Study the drawing (mm; zero at the part's minimum x, y, z) and answer. Coordinates: 2 decimals unless noted, no trailing zeros. Order: outer loops, then holes, each group sorted by start corner. A loop starts at its lowest first (then second) coordinate and runs counter-clockwise, first axis right, second up. Notation, with made-up numbers: (21, -12.5) - (37, -12.5) arc R26 ccw to (37, 6.5) - close; hole circle Ø11 at (-11, 19). An arc over 180 degrees is marked (long way). Write item = value, one per line.
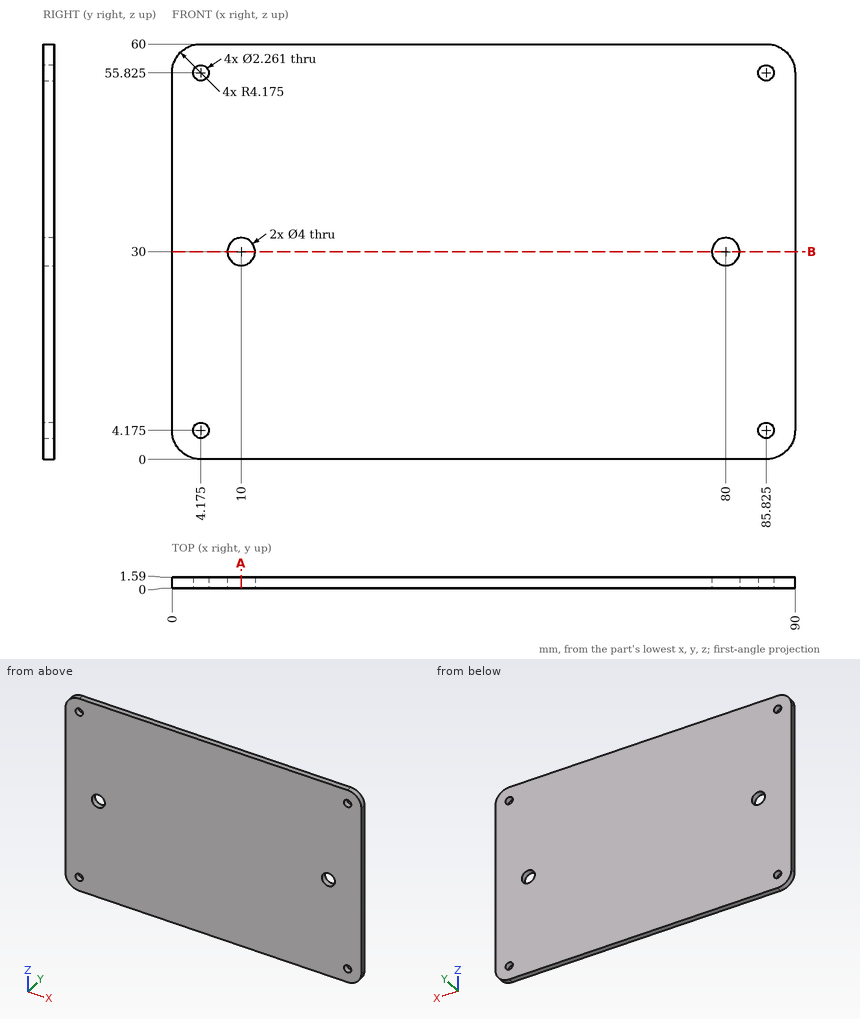
1) Straight lines are drawn through the part: line 1 along X through (y, z) = (0.5, 56); line 2 along X through (y, z) = (1.2, 30); line 3 along Z through (x, y) = (4, 1.2). For each, find the intervals that lie inside material, in ascending order. Write a range as from..to.
Returned:
line_1 = 0..3.06, 5.29..84.71, 86.94..90
line_2 = 0..8, 12..78, 82..90
line_3 = 0..3.06, 5.29..54.71, 56.94..60
2) The part is cut by section A-A (x = 10). Determine the outline of the cut face in (y, z).
Returned:
outline = (0, 0) - (1.59, 0) - (1.59, 28) - (0, 28) - close; (0, 32) - (1.59, 32) - (1.59, 60) - (0, 60) - close
3) A flat-ended cylindrical pin translates along its axis: pin 1 Ø2 at (x, z) = (4.175, 4.175) entering from -Y. Find the tip coordinate at first contact, or state that the pin passes through.
Returned:
pin_1 = through
4) The part is cut by section B-B (z = 30). Determine the outline of the cut face in (x, y).
Returned:
outline = (0, 0) - (8, 0) - (8, 1.59) - (0, 1.59) - close; (12, 0) - (78, 0) - (78, 1.59) - (12, 1.59) - close; (82, 0) - (90, 0) - (90, 1.59) - (82, 1.59) - close
